from build123d import *

# Parameters (mm, degrees)
GRUNDK_RPER_DEPTH               = 100
SCHRAEGEN_VORNE_DEPTH           = 100
SCHNITT_LINEAR_AUSTRAGEN4_DEPTH = 45
WANDUNG1_T                      = -1.75
AUFSATZ_LINEAR_AUSTRAGEN1_DEPTH = 40
AUFSATZ_LINEAR_AUSTRAGEN3_DEPTH = 3
SCHNITT_LINEAR_AUSTRAGEN6_DEPTH = 2.4
SKIZZE13_R                      = 1.7
SCHNITT_LINEAR_AUSTRAGEN7_DEPTH = 2.4


with BuildPart() as part:
    # Skizze1 → Grundkörper (new body)
    with BuildSketch(Plane.XY):
        Polygon((0, 0), (100, 0), (86, 45), (14, 45), align=None)
    extrude(amount=-GRUNDK_RPER_DEPTH)

    # Skizze2 → Schraegen_vorne (cut)
    with BuildSketch(Plane(origin=(0, 0, 0), x_dir=(0, 0, -1), z_dir=(1, 0, 0))):
        Polygon((100, 0), (89, 45), (100, 45), align=None)
    schraegen_vorne = extrude(amount=SCHRAEGEN_VORNE_DEPTH, mode=Mode.SUBTRACT)

    # Spiegel_Schraege_hinten: Schraegen_vorne across plane
    add(schraegen_vorne.mirror(Plane.XY.offset(-50)), mode=Mode.SUBTRACT)

    # Skizze4 → Schnitt-Linear austragen4 (cut)
    with BuildSketch(Plane.XZ):
        with BuildLine():
            Line((5, 0), (95, 0))
            Line((95, 0), (69.229297103, -24.976048727))
            ThreePointArc((69.229297103, -24.976048727), (51.299881289, -33.966183301), (32.533786025, -26.886625433))
            Line((32.533786025, -26.886625433), (5, 0))
        make_face()
    extrude(amount=-SCHNITT_LINEAR_AUSTRAGEN4_DEPTH, mode=Mode.SUBTRACT)

    # Wandung1
    wandung1_openings = [part.faces().sort_by_distance(p)[0] for p in [
        (50.008556747, 0, -58.352640724),
    ]]
    offset(amount=WANDUNG1_T, openings=wandung1_openings, kind=Kind.INTERSECTION)

    # Skizze5 → Aufsatz-Linear austragen1 (add)
    with BuildSketch(Plane.ZY.offset(-27)):
        Polygon((-90.998474583, 9), (-95.998474583, 9), (-96.609585694, 6.5), (-90.998474583, 6.5), align=None)
    extrude(amount=-AUFSATZ_LINEAR_AUSTRAGEN1_DEPTH)

    # Skizze10 → Aufsatz-Linear austragen3 (add)
    with BuildSketch(Plane(origin=(0, 12.75, 0), x_dir=(-1, 0, 0), z_dir=(0, -1, 0))):
        with BuildLine():
            Line((-45, 35.278555896), (-45, 38.999999059))
            ThreePointArc((-45, 38.999999059), (-49.999999529, 44), (-55, 39))
            Line((-55, 39), (-55, 35.278555896))
            ThreePointArc((-55, 35.278555896), (-50, 35.75), (-45, 35.278555896))
        make_face()
    extrude(amount=-AUFSATZ_LINEAR_AUSTRAGEN3_DEPTH)

    # Skizze12 → Schnitt-Linear austragen6 (cut)
    with BuildSketch(Plane.XZ.offset(-12.75)):
        Polygon((46.651368439, -39), (48.325684219, -41.9), (51.674315781, -41.9), (53.348631561, -39), (51.674315781, -36.1), (48.325684219, -36.1), align=None)
    extrude(amount=-SCHNITT_LINEAR_AUSTRAGEN6_DEPTH, mode=Mode.SUBTRACT)

    # Skizze13 → Schnitt-Linear austragen7 (cut)
    with BuildSketch(Plane(origin=(0, 15.75, 0), x_dir=(1, 0, 0), z_dir=(0, 1, 0))):
        with Locations(Location((50, 39, 0), (0, 0, 270))):
            Circle(SKIZZE13_R)
    extrude(amount=-SCHNITT_LINEAR_AUSTRAGEN7_DEPTH, mode=Mode.SUBTRACT)


solid = part.part
Input: part model. Units: mm. Frame: model coordinates. A direction names the side the tool comes from. Give positions to 0.01 mm unless a question says otherwise; leave off trailing zeros. Write each loop counter-clockwise with the first axis right and the second up, starting at its lowest first coordinate (ties: lowest second). Pieces come first, ordered by that corner, then holes.
Q1. Set-up query: faces 3 (the face through (51, 15.75, -41)), 4 (the face through (7.49, 19.06, -4.66)), 5 (the face through (8.655, 21.928, -49.325)). Return all of +Z, -Z, +X, -X, +Y, -Y with unobstructed straight access to the full face (end or side cutting, diameter ignored); none if empty.
Q2. Section C-C, the plane z = -61.5. Output: boundary loops of the cut face in (x, y), plus the area to 3 significant figures.
Q3. Section A-A, the plane x = 50. Output: boundary loops of the cut face in (y, z), plus the area to 3 significant figures.
Q4. Material intervals for probe 1 along X at (y, z) = (34, -11.5); probe 2 along X at (y, z) = (5.5, -25); probe 3 along Y at (x, z) = (79, -42), sorted ascending.
Q5. First-contact query: P1, Ø1, axis at y = 16.5, z = -27.5, coming from the +X side; P2, Ø21, axis at x = 65.5, z = -36.5, coming from the -Y side; P3, Ø3, axis at y = 8, z = -94, coming from the +X side; P4, Ø5, axis at x = 72.5, y = 15.5, coming from the -Z side. Flat tips, straight axial feed; report the tip coordinate or a pass-through.
Q6. Section B-B, the plane y = 35.5. Output: boundary loops of the cut face in (x, z), plus the area to 3 significant figures.
Q7. Pull-direction query (X, two-part tool) for faces 1 (the face through (49.3, 22.18, -94.58)), 2 (the face through (47, 8, -90.998)); classes: pulls with the +X half, pulls with the -X half, needs draft (parallel to the pull), parting line crosses it, or undercut.
Q8. Section D-D, the plane x = 62.5. Output: boundary loops of the cut face in (y, z).
Filled in:
1. face 3: none
1. face 4: +Z, +X, -X, +Y
1. face 5: -Y
2. outline: (0, 0) - (1.83, 0) - (15.29, 43.25) - (84.71, 43.25) - (98.17, 0) - (100, 0) - (86, 45) - (14, 45) - close
2. area: 285 mm2
3. outline: (0, -100) - (45, -89) - (45, -34) - (0, -34) - (0, -35.75) - (12.75, -35.75) - (12.75, -36.1) - (15.15, -36.1) - (15.15, -37.3) - (15.75, -37.3) - (15.75, -35.75) - (43.25, -35.75) - (43.25, -87.63) - (9, -96) - (9, -91) - (6.5, -91) - (6.5, -96.61) - (0, -98.2) - close; (12.75, -44) - (15.75, -44) - (15.75, -40.7) - (15.15, -40.7) - (15.15, -41.9) - (12.75, -41.9) - close
3. area: 272 mm2
4. probe 1: x = 10.58 to 12.41, 14.27 to 16.78, 83.13 to 85.65, 87.59 to 89.42
4. probe 2: x = 1.71 to 3.54, 28.1 to 30.6, 69.21 to 71.72, 96.46 to 98.29
4. probe 3: y = 43.25 to 45
5. P1: stops at x = 95.02
5. P2: stops at y = 0
5. P3: stops at x = 97.98
5. P4: stops at z = -96.82
6. outline: (11.04, -91.32) - (88.96, -91.32) - (88.96, -8.68) - (86.05, -8.68) - (69.23, -24.98) arc R25 cw to (32.53, -26.89) - (13.89, -8.68) - (11.04, -8.68) - close; hole (12.88, -89.52) - (87.12, -89.52) - (87.12, -10.48) - (86.7, -10.48) - (70.51, -26.17) arc R26.75 cw to (31.31, -28.14) - (13.23, -10.48) - (12.88, -10.48) - close
6. area: 599 mm2
7. face 1: needs draft
7. face 2: undercut
8. outline: (0, -100) - (45, -89) - (45, -30.65) - (0, -30.65) - (0, -32.65) - (43.25, -32.65) - (43.25, -87.63) - (9, -96) - (9, -91) - (6.5, -91) - (6.5, -96.61) - (0, -98.2) - close
